Read the model definition and answer for the solid it produces. Units are mm, in the model's axes. A direction names the side the tool comes from. Give positions to 0.01 mm unless a question says otherwise; leave off trailing zeros. Order: outer loops, then holes, each group sorted by start corner. A loop starts at its lowest first (then second) coordinate and runs counter-clockwise, first axis right, second up. Notation, with made-up numbers: (83.25, 55.5) - (128.25, 55.5) arc R15 ccw to (128.25, 59.5) - close; hole circle Ø2 at (12.25, 80.25). An arc over 180 degrees is marked (long way). Return JSON: item names as keys, results as strings.
Autodesk Inventor part; units mm, degrees
ref_plane "YZ Plane" through (0, 0, 0) normal (1, 0, 0) x (0, 1, 0)
ref_plane "XZ Plane" through (0, 0, 0) normal (0, 1, 0) x (-1, 0, 0)
ref_plane "XY Plane" through (0, 0, 0) normal (0, 0, 1) x (1, 0, 0)
sketch "Эскиз1" plane through (0, 0, 0) normal (0, 0, 1) x (1, 0, 0)
  circle A0 centre (0, 0) radius 1.925
  circle A1 centre (0, 0) radius 1.9
  circle A2 centre (0, 0) radius 3.5
  circle A3 centre (0, 0) radius 18.645
  line L0 (0, 69.6007) -> (0, -10.6967)
  circle A4 centre (0, 18.645) radius 1.1
  circle A5 centre (0, 18.645) radius 2
  line L1 (-1.9935, 18.8059) -> (-3.4887, 0.2816)
  line L2 (3.4887, 0.2816) -> (1.9935, 18.8059)
  point P0 (0, 0)
  point P1 (2.0153, 18.5358)
  point P2 (1.9971, 18.5377)
  point P3 (-1.9971, 18.5377)
  point P4 (-2.0153, 18.5358)
  dimension "d0" = 3.8
  dimension "d1" = 7
  dimension "d2" = 2.2
  dimension "d3" = 4
extrude "Выдавливание1" add sketch "Эскиз1" along normal mid plane 2.9 contours A0 L0 A2 | A0 L0 A2 | L0 A5 A3 L2 A2 | A2 L1 A3 A5 L0 | A5 A3 A4 L0 | L0 A4 A3 A5 | A3 A5 L2 | L1 A5 A3 | A5 L0 A4 A3 | A3 A4 L0 A5
sketch "Эскиз2" plane through (0, 0, 1.45) normal (0, 0, 1) x (1, 0, 0)
  line L0 (3.4887, 0.2816) -> (1.9935, 18.8059)
  arc A0 (1.9935, 18.8059) -> (-1.9935, 18.8059) centre (0, 18.645) ccw
  line L1 (-1.9935, 18.8059) -> (-3.4887, 0.2816)
  arc A1 (-3.4887, 0.2816) -> (3.4887, 0.2816) centre (0, 0) ccw
  circle A2 centre (0, 0) radius 1.925
  circle A3 centre (0, 18.645) radius 1.1
  circle A4 centre (0, 0) radius 0.95
  point P0 (0, 0)
  dimension "d8" = 1.9
extrude "Выдавливание2" add sketch "Эскиз2" along normal blind 0.4 contours A1 L1 A0 L0 | A2
properties part number "shatun_main"
Q1. Consider L1, parallel to Y at x = 0, z = -0.1 (3 decimals); L2, parallel to Y at x = 0, z = 1.5 (3 decimals); L3, parallel to X at y = -1, z = 1.1. Determine where each line is inside the solid, lowest interval first.
Values:
{"L1": "y = -3.5 to -1.925, 1.925 to 17.545, 19.745 to 20.645", "L2": "y = -3.5 to -0.95, 0.95 to 17.545, 19.745 to 20.645", "L3": "x = -3.35 to -1.64, 1.64 to 3.35"}
Q2. Given pin 1 (3 mm diameter, centred on x = 0, y = 0, fed in from -Z), flat-ended and moving along its own axis, determine where the tip first touches the part or whether it passes through.
Values:
{"pin 1": "stops at z = 1.45"}
Q3. A cutting plane is placed at C-C (y = 2.5). Write down the section's boundary in (x, z), and give its area (3 significant figures).
Values:
{"outline": "(-3.31, -1.45) - (3.31, -1.45) - (3.31, 1.85) - (-3.31, 1.85) - close", "area": "21.8 mm²"}
Q4. Determine the mould class of faces 1 (the flat face through (2.75, 9.41, 0.18)), 2 (the cylindrical face through (-0.24, 19.72, 0.18)), 3 (the cylindrical face through (-0.1, -3.5, 0)) for opening direction X: released by +X, released by -X, zero draft, split by the parting line, or undercut.
Values:
{"face 1": "released by +X", "face 2": "undercut", "face 3": "split by the parting line"}
Q5. For faces 4 (the cylindrical face through (-0.42, 1.88, -0.02)), 5 (the flat face through (0, 9, -1.45)), determine the directions among +Z, -Z, +X, -X, +Y, -Y from which every point of the face is accessible in a straight line to the end or side of a thin tool.
Values:
{"face 4": "-Z", "face 5": "-Z, +X, -X, +Y, -Y"}
Q6. A cutting plane is placed at A-A (y = 0). Write down the section's boundary in (x, z) (3 decimals).
Values:
{"outline": "(-3.5, -1.45) - (-1.925, -1.45) - (-1.925, 1.45) - (-0.95, 1.45) - (-0.95, 1.85) - (-3.5, 1.85) - close; (0.95, 1.45) - (1.925, 1.45) - (1.925, -1.45) - (3.5, -1.45) - (3.5, 1.85) - (0.95, 1.85) - close"}
Q7. A cutting plane is placed at B-B (x = 0). Write down the section's boundary in (y, z) (3 decimals), and give its area (3 significant figures).
Values:
{"outline": "(-3.5, -1.45) - (-1.925, -1.45) - (-1.925, 1.45) - (-0.95, 1.45) - (-0.95, 1.85) - (-3.5, 1.85) - close; (0.95, 1.45) - (1.925, 1.45) - (1.925, -1.45) - (17.545, -1.45) - (17.545, 1.85) - (0.95, 1.85) - close; (19.745, -1.45) - (20.645, -1.45) - (20.645, 1.85) - (19.745, 1.85) - close", "area": "60.5 mm²"}
Q8. A cutting plane is placed at D-D (y = 19.25). Write down the section's boundary in (x, z).
Values:
{"outline": "(-1.91, -1.45) - (-0.92, -1.45) - (-0.92, 1.85) - (-1.91, 1.85) - close; (0.92, -1.45) - (1.91, -1.45) - (1.91, 1.85) - (0.92, 1.85) - close"}
